from build123d import *

# Parameters (mm, degrees)
F1_DEPTH = 5
F3_D     = 5


with BuildPart() as f1:
    # F0 (on Top) → F1 (new body)
    with BuildSketch(Plane.XY):
        Polygon((107.5, 275), (107.5, 300), (-107.5, 300), (-107.5, 275), (-132.5, 275), (-132.5, -275), (-107.5, -275), (-107.5, -300), (107.5, -300), (107.5, -275), (132.5, -275), (132.5, 275), align=None)
    extrude(amount=F1_DEPTH)

    # F3 (through all)
    with Locations(Plane.XY.offset(5)):
        with Locations((-120, 262.5), (120, 262.5), (-120, -262.5), (120, -262.5)):
            Hole(F3_D / 2)


solid = f1.part
Source: CAD feature listing. Evaluate the final solid. Frame: model axes, mm. Round coordinates to 2 decimals unless told otherwise and drop trailing zeros. Loops run counter-clockwise (first coordinate to the right, second up) from the corner with the lowest first, then second, coordinate; pieces in that order, holes last. Notation, with made-up numbers: M 1,-3.5 L 42,-3.5 A19 cw 42,32.5 Z; hole C 41,7.25 d9. An arc over 180 degrees is marked long. Answer as CSV lines item,"result".
Q1. Contact query for flat-ended pins moving along their axis: pin 1 (1.5 mm diameter, centred on y = -283, z = 3.5, fed in from +X); pin 2 (4.5 mm diameter, centred on x = 120, y = -262.5, fed in from -Z); pin 3 (2.5 mm diameter, centred on x = 122, z = 1.5, fed in from -Y). Output: stop coordinate, or through.
Verdict:
pin 1,"stops at x = 107.5"
pin 2,"passes through"
pin 3,"stops at y = -275"
Q2. Line query: line 1 along Y through (x, z) = (120, 1.6); line 2 along X through (y, z) = (262.5, 3.5); line 3 along Y through (x, z) = (109.5, 1.1). Output: solid intervals per line, ascending.
Verdict:
line 1,"y = -275 to -265, -260 to 260, 265 to 275"
line 2,"x = -132.5 to -122.5, -117.5 to 117.5, 122.5 to 132.5"
line 3,"y = -275 to 275"
Q3. Cut plane A-A (z = 3.55). Return the cut outline in (x, y).
Verdict:
outline,"M -132.5,-275 L -107.5,-275 L -107.5,-300 L 107.5,-300 L 107.5,-275 L 132.5,-275 L 132.5,275 L 107.5,275 L 107.5,300 L -107.5,300 L -107.5,275 L -132.5,275 Z; hole C -120,-262.5 d5; hole C -120,262.5 d5; hole C 120,-262.5 d5; hole C 120,262.5 d5"
